CAD build for the part. Positions are in the model's coordinates, mm. A direction names the side the tool comes from. Give positions to 0.01 mm unless a question says otherwise; leave off trailing zeros. Write each loop counter-clockwise with the first axis right and the second up, starting at its lowest first coordinate (ties: lowest second). Pieces come first, ordered by that corner, then holes. Notation, with made-up numbers: M 70,32.5 L 126,32.5 A17 cw 126,54.5 Z; hole C 76.5,39 d5. An arc over 180 degrees is marked long. One line per question, with ' | ' between items. Start each with the question number.
1. Cut at C-C, the plane x = -16. Write the cut outline in (y, z), then the cut area to 3 significant figures.
2. Which spindle directions (+Z, -Z, +X, -X, +Y, -Y) get a long thin tool onto all of the face, cutting with end or side? Do faces 1 (the face through (23.35, -57.54, -0.74)), 2 (the face through (-4.33, -62.66, 1.48)). Say none if no direction does.
3. Wall check: L1, parallel to Y at x = -50.5, z = 0.15; L2, parallel to Z at x = 29, y = -59; L3, parallel to Y at x = -49.5, z = 1.15. Give the ranges that are in metal, low to high.
4. Flat gauge pin, fed straight in: pin 1 (8 mm diameter, centred on x = 26.5, y = -26, fed in from -Z). Where does the tip first touch, or does it go through?
5. Cut at B-B, the plane y = -81.5. Write the cut outline in (x, z), then the cut area to 3 significant figures.
6. Cut at D-D, the plane y = -41. Write the cut outline in (x, z), then the cut area to 3 significant figures.
7. Pull direction X, two halves, no side cores. Call faces 3 (the face through (-5, 50.687, 1)), 4 (the face through (34.94, -86.45, 1.48)), 5 (the face through (-3.2, -90.586, 1.479)), 6 (the face through (42.92, -97.81, 1.48)): released by +X, released by -X, zero draft, split by the parting line, or undercut.
8. Cut at A-A, the plane x = 15. Write the cut outline in (y, z), then the cut area to 3 significant figures.
Autodesk Inventor part; units mm, degrees
ref_plane "YZ Plane" through (0, 0, 0) normal (1, 0, 0) x (0, 1, 0)
ref_plane "XZ Plane" through (0, 0, 0) normal (0, 1, 0) x (-1, 0, 0)
ref_plane "XY Plane" through (0, 0, 0) normal (0, 0, 1) x (1, 0, 0)
ref_plane "Work Plane1" through (0, 0, 0) normal (0, 0, 1) x (1, 0, 0)
sketch "Sketch1" plane through (0, 0, 0) normal (0, 0, 1) x (1, 0, 0)
  line L0 (39.3474, 50.6868) -> (-50.6526, 50.6868)
  line L1 (-55.6526, 45.6868) -> (-55.6526, -94.3132)
  line L2 (-50.6526, -99.3132) -> (39.3474, -99.3132)
  line L3 (44.3474, -94.3132) -> (44.3474, 45.6868)
  circle A0 centre (15.3748, -79.3757) radius 5.0406
  circle A1 centre (15.3748, -68.2846) radius 2.0418
  arc A2 (44.3474, 45.6868) -> (39.3474, 50.6868) centre (39.3474, 45.6868) ccw
  arc A3 (39.3474, -99.3132) -> (44.3474, -94.3132) centre (39.3474, -94.3132) ccw
  arc A4 (-55.6526, -94.3132) -> (-50.6526, -99.3132) centre (-50.6526, -94.3132) ccw
  arc A5 (-50.6526, 50.6868) -> (-55.6526, 45.6868) centre (-50.6526, 45.6868) ccw
  circle A6 centre (39.3474, 45.6868) radius 1.5
  circle A7 centre (39.3474, -94.3132) radius 1.5
  circle A8 centre (-50.6526, -94.3132) radius 1.5
  circle A9 centre (-50.6526, 45.6868) radius 1.5
  circle A10 centre (-4.0059, -64.1251) radius 1.5
  circle A11 centre (-4.0059, -89.321) radius 1.5
  circle A12 centre (34.2474, -64.1251) radius 1.5
  circle A13 centre (34.2474, -87.7789) radius 1.5
  point P0 (0, 0)
  point P1 (15.2639, -84.621)
  point P2 (44.3474, 50.6868)
  point P3 (-55.6526, -99.3132)
  point P4 (44.3474, -99.3132)
  dimension "d0" = 100
  dimension "d1" = 150
  dimension "d2" = 5
  dimension "d3" = 3
  dimension "d4" = 3
  dimension "d5" = 3
  dimension "d6" = 3
  dimension "d7" = 3
  dimension "d8" = 3
  dimension "d9" = 3
  dimension "d10" = 3
extrude "Extrusion1" add sketch "Sketch1" along normal blind 3
sketch "Sketch2" plane through (0, 0, 0) normal (0, 0, -1) x (-1, 0, 0)
  circle A0 centre (-6.6801, -58.8323) radius 1.4403
  circle A1 centre (-24.0209, -58.8323) radius 1.4576
  point P0 (0, 0)
extrude "Extrusion2" add sketch "Sketch2" along normal blind 1.5
properties part number "TopPlate" material "Glass"
Here are the results:
1) outline: M -99.31,0 L 50.69,0 L 50.69,3 L -99.31,3 Z | area: 450 mm^2
2) face 1: -Z | face 2: +Z, -Z
3) L1: -99.31 to -95.81, -92.82 to 44.19, 47.18 to 50.69 | L2: 0 to 3 | L3: -99.31 to -95.27, -93.35 to 44.73, 46.65 to 50.69
4) pin 1: z = 0
5) outline: M -55.65,0 L 10.8,0 L 10.8,3 L -55.65,3 Z; M 19.95,0 L 44.35,0 L 44.35,3 L 19.95,3 Z | area: 273 mm^2
6) outline: M -55.65,0 L 44.35,0 L 44.35,3 L -55.65,3 Z | area: 300 mm^2
7) face 3: zero draft | face 4: undercut | face 5: undercut | face 6: released by +X
8) outline: M -99.31,0 L -84.4,0 L -84.4,3 L -99.31,3 Z; M -74.35,0 L -70.29,0 L -70.29,3 L -74.35,3 Z; M -66.28,0 L 50.69,0 L 50.69,3 L -66.28,3 Z | area: 408 mm^2
